Here's the drawing with two shaded views (mm, measured from the low corner). I have some questions. Coordinates: 2 decimals unless noted, no trailing zeros. Loops run counter-clockwise (first coordinate to the right, second up) from the corner with the lowest first, then second, coordinate; pieces in that order, holes last.
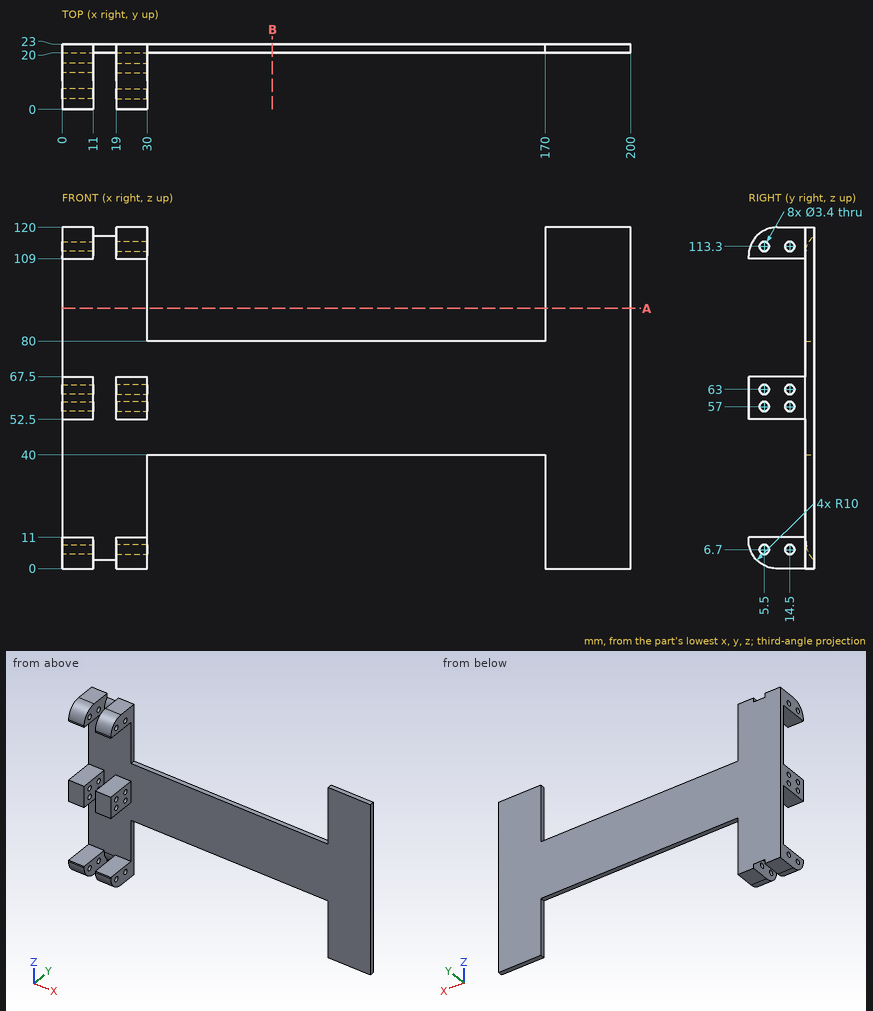
(1) I want a section at B-B on x = 74. Write out the boundary of the cut face in (y, z), then the cut area to 3 significant figures.
Check values:
outline: (20, 40) - (23, 40) - (23, 80) - (20, 80) - close
area: 120 mm2
(2) I'm going to push flat-ended pins straight in: pin 1 (3.5 mm diameter, centred on x = 3, y = 8, fed in from +Z); pin 2 (0.9 mm diameter, centred on x = 115, y = 22, fed in from -Z); pin 3 (4.5 mm diameter, centred on y = 14.5, z = 57, fed in from +X). Where does each tip first touch, or does it pass through?
Check values:
pin 1: stops at z = 120
pin 2: stops at z = 40
pin 3: stops at x = 30
(3) I want a section at A-A on z = 91.5. Write out the boundary of the cut face in (x, y), then the cut area to 3 significant figures.
Check values:
outline: (0, 20) - (30, 20) - (30, 23) - (0, 23) - close; (170, 20) - (200, 20) - (200, 23) - (170, 23) - close
area: 180 mm2
(4) If I drill on probe 1 along Y at (x, z) = (27.75, 63); probe 2 along Y at (x, z) = (6.5, 6.7); probe 3 along X at (y, z) = (22, 10), over which ranges is the centre line in solid material (lowest first)?
Check values:
probe 1: y = 0 to 3.8, 7.2 to 12.8, 16.2 to 23
probe 2: y = 0.56 to 3.8, 7.2 to 12.8, 16.2 to 23
probe 3: x = 0 to 30, 170 to 200
